from build123d import *

# Parameters (mm, degrees)
SKETCH1_W           = 126
SKETCH1_H           = 115
BOSS_EXTRUDE1_DEPTH = 2
SKETCH2_R           = 7.5
SKETCH2_W           = 60
SKETCH2_H           = 25
CUT_EXTRUDE1_DEPTH  = 2
FILLET1_R           = 3
SKETCH3_R           = 1.3
CUT_EXTRUDE2_DEPTH  = 4
SKETCH4_W           = 3
SKETCH4_H           = 6
SKETCH4_H_2         = 1.5
CUT_EXTRUDE3_DEPTH  = 10
FILLET2_R           = 1
SKETCH6_W           = 15
SKETCH6_H           = 10
SKETCH6_W_2         = 16.5
SKETCH6_H_2         = 8
CUT_EXTRUDE5_DEPTH  = 10
FILLET3_R           = 1
SKETCH7_R           = 1.3
CUT_EXTRUDE6_DEPTH  = 2.5


with BuildPart() as part:
    # Sketch1 → Boss-Extrude1 (new body)
    with BuildSketch(Plane.XY):
        Rectangle(SKETCH1_W, SKETCH1_H)
    extrude(amount=BOSS_EXTRUDE1_DEPTH)

    # Sketch2 → Cut-Extrude1 (cut)
    with BuildSketch(Plane.XY.offset(2)):
        with Locations((-43, -40)):
            Circle(SKETCH2_R)
        with Locations((43, -40)):
            Circle(SKETCH2_R)
        with Locations((0, -37)):
            Rectangle(SKETCH2_W, SKETCH2_H)
    extrude(amount=-CUT_EXTRUDE1_DEPTH, mode=Mode.SUBTRACT)

    # Fillet1
    fillet1_edges = [part.edges().sort_by_distance(p)[0] for p in [
        (30, -24.5, 1),
        (30, -49.5, 1),
        (-30, -49.5, 1),
        (-30, -24.5, 1),
    ]]
    fillet(fillet1_edges, radius=FILLET1_R)

    # Sketch3 → Cut-Extrude2 (cut)
    with BuildSketch(Plane.XY.offset(2)):
        with Locations((-26, 47.5)):
            Circle(SKETCH3_R)
        with Locations((-36, 47.5)):
            Circle(SKETCH3_R)
        with Locations((36, 47.5)):
            Circle(SKETCH3_R)
        with Locations((26, 47.5)):
            Circle(SKETCH3_R)
        with Locations((-26, 37.5)):
            Circle(SKETCH3_R)
        with Locations((-36, 37.5)):
            Circle(SKETCH3_R)
        with Locations((36, 37.5)):
            Circle(SKETCH3_R)
        with Locations((26, 37.5)):
            Circle(SKETCH3_R)
    extrude(amount=-CUT_EXTRUDE2_DEPTH, mode=Mode.SUBTRACT)

    # Sketch4 → Cut-Extrude3 (cut)
    with BuildSketch(Plane(origin=(0, 0, 0), x_dir=(-1, 0, 0), z_dir=(0, 0, -1))):
        with Locations((-31, 54.5)):
            Rectangle(SKETCH4_W, SKETCH4_H)
        with Locations((31, 54.5)):
            Rectangle(SKETCH4_W, SKETCH4_H)
        with Locations((31, -56.75)):
            Rectangle(SKETCH4_W, SKETCH4_H_2)
        with Locations((-31, -56.75)):
            Rectangle(SKETCH4_W, SKETCH4_H_2)
    extrude(amount=-CUT_EXTRUDE3_DEPTH, mode=Mode.SUBTRACT)

    # Fillet2
    fillet2_edges = [part.edges().sort_by_distance(p)[0] for p in [
        (-29.5, -57.5, 1),
        (-32.5, -57.5, 1),
        (29.5, -57.5, 1),
        (32.5, -57.5, 1),
        (29.5, 57.5, 1),
        (32.5, 57.5, 1),
        (-32.5, 57.5, 1),
        (-29.5, 57.5, 1),
        (63, -57.5, 1),
        (-63, -57.5, 1),
        (-63, 57.5, 1),
        (63, 57.5, 1),
    ]]
    fillet(fillet2_edges, radius=FILLET2_R)

    # Sketch6 → Cut-Extrude5 (cut)
    with BuildSketch(Plane.XY.offset(2)):
        with Locations((20, 0)):
            Rectangle(SKETCH6_W, SKETCH6_H)
        with BuildLine():
            Line((4.472135955, 4), (-4.472135955, 4))
            ThreePointArc((-4.472135955, 4), (-6, 0), (-4.472135955, -4))
            Line((-4.472135955, -4), (4.472135955, -4))
            ThreePointArc((4.472135955, -4), (5.605034154, -2.140932539), (6, 0))
            ThreePointArc((6, 0), (5.605034154, 2.140932539), (4.472135955, 4))
        make_face()
        with BuildLine():
            Line((8.25, 4), (4.472135955, 4))
            ThreePointArc((4.472135955, 4), (5.605034154, 2.140932539), (6, 0))
            ThreePointArc((6, 0), (5.605034154, -2.140932539), (4.472135955, -4))
            Line((4.472135955, -4), (8.25, -4))
            Line((8.25, -4), (8.25, 4))
        make_face()
        with BuildLine():
            ThreePointArc((4.472135955, 4), (0, 6), (-4.472135955, 4))
            Line((-4.472135955, 4), (4.472135955, 4))
        make_face()
        with BuildLine():
            Line((-4.472135955, 4), (-8.25, 4))
            Line((-8.25, 4), (-8.25, -4))
            Line((-8.25, -4), (-4.472135955, -4))
            ThreePointArc((-4.472135955, -4), (-6, 0), (-4.472135955, 4))
        make_face()
        with BuildLine():
            Line((4.472135955, -4), (-4.472135955, -4))
            ThreePointArc((-4.472135955, -4), (0, -6), (4.472135955, -4))
        make_face()
        with Locations((-20, 0)):
            Rectangle(SKETCH6_W_2, SKETCH6_H_2)
    extrude(amount=-CUT_EXTRUDE5_DEPTH, mode=Mode.SUBTRACT)

    # Fillet3
    fillet3_edges = [part.edges().sort_by_distance(p)[0] for p in [
        (27.5, 5, 1),
        (27.5, -5, 1),
        (12.5, -5, 1),
        (12.5, 5, 1),
        (4.472135955, 4, 1),
        (8.25, 4, 1),
        (8.25, -4, 1),
        (4.472135955, -4, 1),
        (-4.472135955, -4, 1),
        (-8.25, -4, 1),
        (-8.25, 4, 1),
        (-4.472135955, 4, 1),
        (-11.75, 4, 1),
        (-11.75, -4, 1),
        (-28.25, -4, 1),
        (-28.25, 4, 1),
    ]]
    fillet(fillet3_edges, radius=FILLET3_R)

    # Sketch7 → Cut-Extrude6 (cut)
    with BuildSketch(Plane(origin=(0, 0, 0), x_dir=(-1, 0, 0), z_dir=(0, 0, -1))):
        with Locations((-50, -17)):
            Circle(SKETCH7_R)
        with Locations((-20, -17)):
            Circle(SKETCH7_R)
        with Locations((20, -17)):
            Circle(SKETCH7_R)
        with Locations((50, -17)):
            Circle(SKETCH7_R)
    extrude(amount=-CUT_EXTRUDE6_DEPTH, mode=Mode.SUBTRACT)


solid = part.part
Work out the finished part from the listing and answer in its coordinate system (mm). A direction names the side the tool comes from. Give positions to 0.01 mm unless a question says otherwise; leave off trailing zeros. Loops run counter-clockwise (first coordinate to the right, second up) from the corner with the lowest first, then second, coordinate; pieces in that order, holes last. Notation, with made-up numbers: (65.5, 57) -> (101.5, 57) arc R6 cw to (101.5, 68) -> close; hole circle Ø1 at (-15, 12). An arc over 180 degrees is marked (long way). Use a Markdown table: item, result. Add a question column.
1. Section C-C on x = -15 is taken. Determine the outline of the cut face in (y, z), and give its area (3 significant figures).
2. Section A-A on y = -40 is taken. Determine the outline of the cut face in (x, z), and give its area (3 significant figures).
3. Flat-ended cylindrical pins translate along their axes: pin 1 Ø6 at (x, y) = (-43.5, 26.5) entering from -Z; pin 2 Ø0.6 at (x, z) = (-31.5, 1) entering from -Y; pin 3 Ø2.5 at (x, y) = (36, 47.5) entering from +Z. Find the tip coordinate at first contact, or state that the pin passes through.
4. For faces 1 (the cylindrical face through (29.1, -48.64, 0.99)), 2 (the flat face through (-1, 14, 0)), determine the directions among +Z, -Z, +X, -X, +Y, -Y from which every point of the face is accessible in a straight line to the end or side of a thin tool.
5. Find the intervals of material crossed by probe 1 along Y at (x, z) = (24, 1.55); probe 2 along Y at (x, z) = (-16.5, 0.1); probe 3 along Y at (x, z) = (-26, 1.1), in increasing order.
6. Section D-D on z = 1 is taken. State how many separate pieces and enclosed holes the cut face has, and give its area (3 significant figures).
7. Determine the mould class of faces 3 (the cylindrical face through (51.3, -16.94, 0.99)), 4 (the flat face through (-1, 14, 2)) for opening direction Y: released by +Y, released by -Y, zero draft, split by the parting line, or undercut.
8. Section B-B on x = 43 is taken. Determine the outline of the cut face in (y, z), and give its area (3 significant figures).
Results below:
| question | item | result |
|---|---|---|
| 1 | outline | (-57.5, 0) -> (-49.5, 0) -> (-49.5, 2) -> (-57.5, 2) -> close; (-24.5, 0) -> (-4, 0) -> (-4, 2) -> (-24.5, 2) -> close; (4, 0) -> (57.5, 0) -> (57.5, 2) -> (4, 2) -> close |
| 1 | area | 164 mm^2 |
| 2 | outline | (-63, 0) -> (-50.5, 0) -> (-50.5, 2) -> (-63, 2) -> close; (-35.5, 0) -> (-30, 0) -> (-30, 2) -> (-35.5, 2) -> close; (30, 0) -> (35.5, 0) -> (35.5, 2) -> (30, 2) -> close; (50.5, 0) -> (63, 0) -> (63, 2) -> (50.5, 2) -> close |
| 2 | area | 72.0 mm^2 |
| 3 | pin 1 | stops at z = 0 |
| 3 | pin 2 | stops at y = -56 |
| 3 | pin 3 | passes through |
| 4 | face 1 | +Z, -Z |
| 4 | face 2 | -Z, +X, -X, +Y, -Y |
| 5 | probe 1 | y = -57.5 to -49.5, -24.5 to -5, 5 to 57.5 |
| 5 | probe 2 | y = -57.5 to -49.5, -24.5 to -4, 4 to 57.5 |
| 5 | probe 3 | y = -57.5 to -49.5, -24.5 to -4, 4 to 36.2, 38.8 to 46.2, 48.8 to 57.5 |
| 6 | separate pieces | 1 |
| 6 | enclosed holes | 18 |
| 6 | area | 12,100 mm^2 |
| 7 | face 3 | undercut |
| 7 | face 4 | zero draft |
| 8 | outline | (-57.5, 0) -> (-47.5, 0) -> (-47.5, 2) -> (-57.5, 2) -> close; (-32.5, 0) -> (57.5, 0) -> (57.5, 2) -> (-32.5, 2) -> close |
| 8 | area | 200 mm^2 |
